Could you check a few things on this model? Use its own coordinates, in mm. A direction names the side the tool comes from. Round coordinates to 2 decimals unless told otherwise and drop trailing zeros. Write each loop counter-clockwise with the first axis right and the second up, starting at its lowest first coordinate (ties: lowest second). Pieces come first, ordered by that corner, then holes. Notation, with made-up numbers: M 20,-1 L 68,-1 A18 cw 68,15 Z; hole C 47.25,-6.75 d10. An arc over 180 degrees is marked long. One line per item, written item: value. Start each with the question number.
(1) I'm going to push flat-ended pins straight in: pin 1 Ø5 at (x, y) = (-28.5, 8.5) entering from +Z; pin 2 Ø7.5 at (x, y) = (-65, 10.25) entering from +Z. Where does each tip first touch, or does it pass through?
(2) Which directions (+Z, -Z, +X, -X, +Y, -Y) give clear straight access to the entire face, cutting with the end or side of a thin tool? Please do faces 5 (the face through (-62.85, 10.34, 1.48)), 6 (the face through (-67, 8, 3)).
(3) I want a section at B-B on x = -51.5. Please give me the cut outline in (y, z).
(4) I want a section at A-A on y = 10.25. Please give me the cut outline in (x, z).
(5) Thinking about a two-plate mould opening in Y: for faces 1 (the face through (1.05, 13.597, 4.007)), 2 (the face through (-75, 8, 2)), 3 (the face through (64.447, 6.036, 3.764)), 4 (the face through (1, 0, 2)), which applies, released by +Y, released by -Y, zero draft, split by the parting line, or undercut?
(6) If I drill on L1, parallel to X at y = 10.25, z = 3.6; L2, parallel to Y at x = 65, z = 0.95; L3, parallel to X at y = 8.75, z = 2.35, over which ranges is the centre line in solid material (lowest first)?
(7) I want a section at C-C on z = 3.8. Please give me the cut outline in (x, y).
Autodesk Inventor part; units mm, degrees
ref_plane "YZ Plane" through (0, 0, 0) normal (1, 0, 0) x (0, 1, 0)
ref_plane "XZ Plane" through (0, 0, 0) normal (0, 1, 0) x (-1, 0, 0)
ref_plane "XY Plane" through (0, 0, 0) normal (0, 0, 1) x (1, 0, 0)
sketch "スケッチ1" plane through (0, 0, 0) normal (0, 0, 1) x (1, 0, 0)
  line L0 (-75, 20.5) -> (75, 20.5)
  line L1 (75, 20.5) -> (75, 0)
  line L2 (75, 0) -> (-75, 0)
  line L3 (-75, 0) -> (-75, 20.5)
  circle A0 centre (-65, 10.25) radius 4.25
  circle A1 centre (65, 10.25) radius 4.25
  point P0 (0, 0)
  point P1 (0, 0)
  dimension "d0" = 20.5
  dimension "d1" = 150
  dimension "d2" = 10.25
  dimension "d3" = 130
  dimension "d4" = 10
  dimension "d5" = 8.5
extrude "押し出し1" add sketch "スケッチ1" along normal blind 5
sketch "スケッチ3" plane through (75, 0, 0) normal (1, 0, 0) x (0, 0, -1)
  line L0 (0, 0) -> (0, 20.5) construction
  line L1 (0, 20.5) -> (-5, 20.5) construction
  line L2 (-5, 0) -> (-5, 20.5) construction
  line L3 (0, 0) -> (-5, 0) construction
  line L4 (0, 20.5) -> (-5, 20.5)
  arc A0 (-1.2, 20.5) -> (-5, 6) centre (24.5645, 6) ccw
  line L5 (-5, 0) -> (-5, 20.5)
  line L6 (-1.2, 20.5) -> (-5, 13.7479) construction
  line L7 (-1.2, 20.5) -> (-5, 20.5)
  line L8 (-5, 6) -> (-5, 20.5)
  point P0 (0, 0)
  dimension "d12" = 1.2
  dimension "d13" = 6
extrude "押し出し3" cut sketch "スケッチ3" against normal through all
sketch "スケッチ4" plane through (0, 0, 0) normal (0, 0, -1) x (-1, 0, 0)
  circle A0 centre (-65, 10.25) radius 4.25
  circle A1 centre (65, 10.25) radius 4.25
  circle A2 centre (-65, 10.25) radius 2.15
  circle A3 centre (65, 10.25) radius 2.15
  point P0 (0, 0)
  dimension "d16" = 4.3
extrude "押し出し4" add sketch "スケッチ4" against normal blind 3
equation "\"d2\" = 0.5 * d0"
equation "\"d4\" = -0.5 * d3 + 0.5 * d1"
properties part number "top_140mm_2"
Found:
1. pin 1: stops at z = 5
1. pin 2: stops at z = 3
2. face 5: +Z, -Z
2. face 6: +Z
3. outline: M 0,0 L 20.5,0 L 20.5,1.2 A29.56 ccw 6,5 L 0,5 Z
4. outline: M -75,0 L -67.15,0 L -67.15,3 L -69.25,3 L -69.25,4.69 L -75,4.69 Z; M -62.85,0 L 62.85,0 L 62.85,3 L 60.75,3 L 60.75,4.69 L -60.75,4.69 L -60.75,3 L -62.85,3 Z; M 67.15,0 L 75,0 L 75,4.69 L 69.25,4.69 L 69.25,3 L 67.15,3 Z
5. face 1: released by +Y
5. face 2: zero draft
5. face 3: undercut
5. face 4: released by -Y
6. L1: x = -75 to -69.25, -60.75 to 60.75, 69.25 to 75
6. L2: y = 0 to 8.1, 12.4 to 20.5
6. L3: x = -75 to -66.54, -63.46 to 63.46, 66.54 to 75
7. outline: M -75,0 L 75,0 L 75,14.34 L 66.16,14.34 A4.25 cw long 63.84,14.34 L -63.84,14.34 A4.25 cw long -66.16,14.34 L -75,14.34 Z
